For this review, take the finished solid that the model builds, in its own axes (mm). Face numbers are marked on the shaded views. A direction names the side the tool comes from. Coordinates: 2 decimals unless noted, no trailing zeros. Write each loop counter-clockwise with the first axis right and the second up, starting at its lowest first coordinate (ties: lowest second). Pieces come first, ordered by that corner, then holes.
```python
from build123d import *

# Parameters (mm, degrees)
BOSS_EXTRUDE1_DEPTH     = 9.525
SKETCH2_3_W             = 49.295937228
SKETCH2_3_H             = 6.35
BOSS_EXTRUDE2_DEPTH     = 15.875
SKETCH10_W              = 19.05
SKETCH10_H              = 6.35
CUT_EXTRUDE1_DEPTH      = 45.031748726
CUT_EXTRUDE1_DEPTH_BACK = 45.031748726
CUT_EXTRUDE2_DEPTH      = 45.031748726
CUT_EXTRUDE2_DEPTH_BACK = 45.031748726
CUT_EXTRUDE3_REACH      = 62.033
SKETCH14_R              = 2.5527
CUT_EXTRUDE4_DEPTH      = 45.031748726
FILLET1_R               = 3.175
SKETCH17_W              = 3.96875
SKETCH17_H              = 3.175
CUT_EXTRUDE5_DEPTH      = 59.036347156


with BuildPart() as part:
    # Sketch2 → Boss-Extrude1 (new, symmetric)
    with BuildSketch(Plane(origin=(0, 0, 0), x_dir=(1, 0, 0), z_dir=(0, 1, 0))):
        Polygon((24.647968614, 26.19375), (-24.647968614, 26.19375), (1.931794404, -19.84375), (24.647968614, -19.84375), align=None)
    extrude(amount=BOSS_EXTRUDE1_DEPTH, both=True)

    # Sketch2<3> → Boss-Extrude2 (add, symmetric)
    with BuildSketch(Plane(origin=(0, 0, 0), x_dir=(1, 0, 0), z_dir=(0, 1, 0))):
        with Locations((0, -23.01875)):
            Rectangle(SKETCH2_3_W, SKETCH2_3_H)
    extrude(amount=BOSS_EXTRUDE2_DEPTH, both=True)

    # Cut-Sweep1: sweep along a curve in space
    with BuildLine() as cut_sweep1_path:
        Line((-24.647968614, 9.525, -26.19375), (1.931794404, 9.525, 19.84375))
    # Sketch10 → Cut-Sweep1 (sweep, cut)
    with BuildSketch(Plane(origin=(0, 0, -26.19375), x_dir=(-1, 0, 0), z_dir=(0, 0, -1))):
        with Locations((15.122968614, 0)):
            Rectangle(SKETCH10_W, SKETCH10_H)
    sweep(path=cut_sweep1_path.line, mode=Mode.SUBTRACT)

    # Sketch11 → Cut-Extrude1 (cut, two sides: drawn at the far end of the back side and taken through both)
    with BuildSketch(Plane(origin=(0, 9.525, 0), x_dir=(1, 0, 0), z_dir=(0, 1, 0)).offset(-CUT_EXTRUDE1_DEPTH_BACK)):
        Polygon((-19.885468614, 26.19375), (-24.647968614, 26.19375), (-19.885468614, 17.944858029), align=None)
    extrude(amount=CUT_EXTRUDE1_DEPTH + CUT_EXTRUDE1_DEPTH_BACK, mode=Mode.SUBTRACT)

    # Sketch13 → Cut-Extrude2 (cut, two sides: drawn at the far end of the back side and taken through both)
    with BuildSketch(Plane(origin=(0, 9.525, 0), x_dir=(1, 0, 0), z_dir=(0, 1, 0)).offset(-CUT_EXTRUDE2_DEPTH_BACK)):
        Polygon((-13.649445986, 19.84375), (9.264142823, -19.84375), (15.423315495, -19.84375), (-7.490273314, 19.84375), align=None)
    extrude(amount=CUT_EXTRUDE2_DEPTH + CUT_EXTRUDE2_DEPTH_BACK, mode=Mode.SUBTRACT)

    # Sketch14 → Cut-Extrude3 (cut, up to next)
    with BuildSketch(Plane.XY.offset(26.19375), mode=Mode.PRIVATE) as cut_extrude3_sk1:
        with Locations((10.277031386, 0)):
            Circle(SKETCH14_R)
    cut_extrude3_tool1 = extrude(cut_extrude3_sk1.sketch, amount=-CUT_EXTRUDE3_REACH, mode=Mode.PRIVATE) & part.part
    # Sketch14 → Cut-Extrude3 (cut, up to next)
    with BuildSketch(Plane.XY.offset(26.19375), mode=Mode.PRIVATE) as cut_extrude3_sk2:
        with Locations((-5.597968614, 0)):
            Circle(SKETCH14_R)
    cut_extrude3_tool2 = extrude(cut_extrude3_sk2.sketch, amount=-CUT_EXTRUDE3_REACH, mode=Mode.PRIVATE) & part.part
    add(cut_extrude3_tool1.solids().sort_by_distance((10.277031, 0, 26.19375))[0], mode=Mode.SUBTRACT)
    add(cut_extrude3_tool2.solids().sort_by_distance((-5.597969, 0, 26.19375))[0], mode=Mode.SUBTRACT)

    # Sketch16 → Cut-Extrude4 (cut, through all)
    with BuildSketch(Plane(origin=(0, 9.525, 0), x_dir=(1, 0, 0), z_dir=(0, 1, 0))):
        Polygon((-0.157924895, 19.84375), (19.567968614, -14.322499782), (19.567968614, 19.84375), align=None)
    extrude(amount=-CUT_EXTRUDE4_DEPTH, mode=Mode.SUBTRACT)

    # Fillet1
    fillet1_edges = [part.edges().sort_by_distance(p)[0] for p in [
        (-0.157924895, 0, -19.84375),
        (19.567968614, 0, -19.84375),
        (19.567968614, 0, 14.322499782),
    ]]
    fillet(fillet1_edges, radius=FILLET1_R)

    # Sketch17 → Cut-Extrude5 (cut, through all)
    with BuildSketch(Plane(origin=(24.647968614, 0, 0), x_dir=(0, 0, -1), z_dir=(1, 0, 0))):
        with Locations((22.225, 7.9375)):
            Rectangle(SKETCH17_W, SKETCH17_H)
        with Locations((22.225, -7.9375)):
            Rectangle(SKETCH17_W, SKETCH17_H)
    extrude(amount=-CUT_EXTRUDE5_DEPTH, mode=Mode.SUBTRACT)


solid = part.part
```
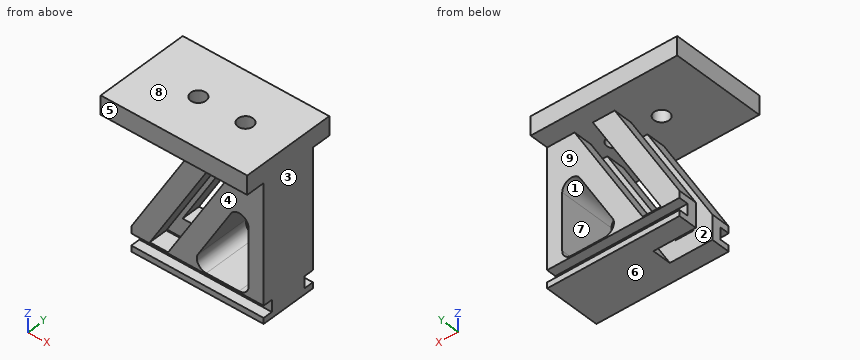
Q1. Add section D-D (x = 1). State the section outline as (y, z) points (3 decimals), then the cut area to 3 significant figures.
Ans:
outline: (-15.875, 19.844) - (15.875, 19.844) - (15.875, 26.194) - (-15.875, 26.194) - close; (-9.525, -26.194) - (9.525, -26.194) - (9.525, -24.209) - (6.35, -24.209) - (6.35, -20.241) - (9.525, -20.241) - (9.525, -5.138) - (3.175, -5.138) - (3.175, -14.766) - (-3.175, -14.766) - (-3.175, -5.138) - (-9.525, -5.138) - (-9.525, -20.241) - (-6.35, -20.241) - (-6.35, -24.209) - (-9.525, -24.209) - close; (-9.525, 5.53) - (-3.175, 5.53) - (-3.175, 18.23) - (-9.525, 18.23) - close; (3.175, 5.53) - (9.525, 5.53) - (9.525, 18.23) - (3.175, 18.23) - close
area: 678 mm2
Q2. Tool access review of the marked faces 1, 2, 3, 4 and 5: name each direction out of +Z, -Z, +X, -X, +Y, -Y from which nothing blocks a thin tool from reaching the whole face with its end or side.
Ans:
face 1: +Y, -Y
face 2: -X
face 3: +Z, -Z, +X, +Y, -Y
face 4: -Z, +X, -X, -Y
face 5: +Z, -Z, +X, -X, -Y
Q3. For probe 1 along Y at (x, z) = (-2, 6) (3 decimals); probe 2 along Z at (x, y) = (15, 6.5); probe 3 along X at (y, z) = (-2, 23.5), list the stretches that pass through material, from the lowest coordinate up.
Ans:
probe 1: y = -9.525 to -3.175, 3.175 to 9.525
probe 2: z = -26.19 to -24.21, -20.24 to -19.84, 5.33 to 19.11, 19.84 to 26.19
probe 3: x = -24.65 to -7.18, -4.01 to 8.69, 11.86 to 24.65
Q4. Add section B-B (z = 17.5). State the section outline as (x, y) points (3 decimals).
Ans:
outline: (0.579, -9.525) - (7.911, -9.525) - (7.911, -3.175) - (0.579, -3.175) - close; (0.579, 3.175) - (7.911, 3.175) - (7.911, 9.525) - (0.579, 9.525) - close; (14.07, -9.525) - (24.648, -9.525) - (24.648, 9.525) - (14.07, 9.525) - (14.07, 3.175) - (19.629, 3.175) - (19.629, -3.175) - (14.07, -3.175) - close
Q5. Add section C-C (y = 5). State the section outline as (x, z) points (3 decimals), then the cut area to 3 significant figures.
Ans:
outline: (-24.648, 19.844) - (1.932, 19.844) - (-19.885, -17.945) - (-19.885, -26.194) - (24.648, -26.194) - (24.648, 26.194) - (-24.648, 26.194) - close; hole (-13.649, -19.844) - (-7.49, -19.844) - (15.423, 19.844) - (9.264, 19.844) - close; hole (2.592, -15.081) arc R3.175 ccw to (5.341, -19.844) - (16.393, -19.844) arc R3.175 ccw to (19.568, -16.669) - (19.568, 2.473) arc R3.175 ccw to (13.643, 4.061) - close
area: 1,400 mm2
Q6. Clearance check with flat-ended pins moving along their axes: pin 1 Ø5 at (y, z) = (7, -23) entering from -X; pin 2 Ø2 at (y, z) = (-2, -17.5) entering from -X; pin 3 Ø20 at (x, z) = (7, -7) entering from -Y (3 decimals); pin 4 Ø6 at (x, y) = (10.28, 0) entering from +Z. State where each tip first meets the part, or that it passes through.
Ans:
pin 1: stops at x = -19.89
pin 2: stops at x = -1.16
pin 3: stops at y = -9.525
pin 4: stops at z = 26.19
Q7. Add section A-A (y = 0). State the section outline as (x, z) points (3 decimals).
Ans:
outline: (-24.648, 19.844) - (-8.151, 19.844) - (-8.151, 26.194) - (-24.648, 26.194) - close; (-5.598, -26.194) - (24.648, -26.194) - (24.648, 26.194) - (12.83, 26.194) - (12.83, 19.844) - (20.982, 19.844) - close; (-3.045, 19.844) - (7.724, 19.844) - (7.724, 26.194) - (-3.045, 26.194) - close; hole (2.592, -15.081) arc R3.175 ccw to (5.341, -19.844) - (16.393, -19.844) arc R3.175 ccw to (19.568, -16.669) - (19.568, 2.473) arc R3.175 ccw to (13.643, 4.061) - close
Q8. Draft analysis for pull direction Z (two halves, no side actions). For the marked faces 6, 7, 8 and 9, state which applies: +Z half, -Z half, draft (parallel to the pull), parting line (faces both ways), or undercut.
Ans:
face 6: -Z half
face 7: undercut
face 8: +Z half
face 9: draft
